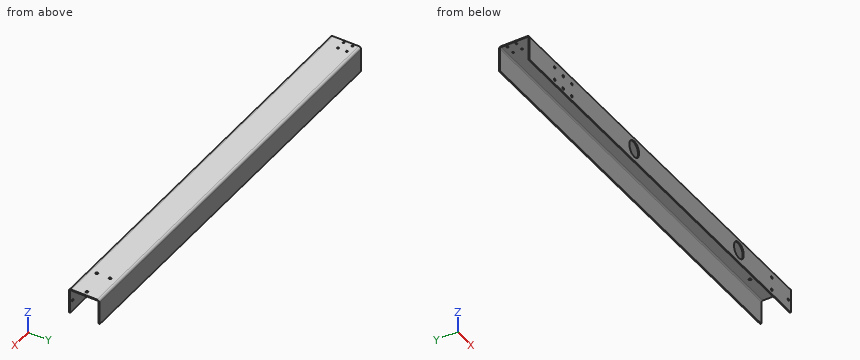
```python
from build123d import *

# Parameters (mm, degrees)
SKETCH1_W                           = 1203.325
SKETCH1_H                           = 74.6125
BASE_FLANGE1_DEPTH                  = 3.175
EDGE_FLANGE1_STRIP_W                = 20.32
EDGE_FLANGE1_STRIP_H                = 3.175
EDGE_FLANGE1_STRIP_CUT_DEPTH        = 1203.325
EDGE_FLANGE1_DEPTH                  = 1203.325
EDGE_FLANGE2_STRIP_W                = 20.32
EDGE_FLANGE2_STRIP_H                = 3.175
EDGE_FLANGE2_STRIP_CUT_DEPTH        = 1203.325
EDGE_FLANGE2_DEPTH                  = 1203.325
F_9_32_0_28125_DIAMETER_HOLE3_D     = 7.14375
F_9_32_0_28125_DIAMETER_HOLE3_DEPTH = 3.175
FILLET1_R                           = 3.175
F_9_32_0_28125_DIAMETER_HOLE1_D     = 7.14375
F_9_32_0_28125_DIAMETER_HOLE1_DEPTH = 3.175
F_9_32_0_28125_DIAMETER_HOLE2_D     = 7.14375
F_1_1_71_DOWEL_SLOT1_DEPTH          = 3.175
F_10_0_1935_DIAMETER_HOLE1_D        = 4.9149
LPATTERN2_COUNT                     = 2
LPATTERN2_PITCH                     = 25.4
LPATTERN2_COUNT_DIR2                = 2
LPATTERN2_PITCH_DIR2                = 25.4


# Read off the part's stored shape, not the designer's step: 1 (1.71) Dowel Slot1
# Sheet-metal steps are written as plain solids
with BuildPart() as part:
    # Sketch1 → Base-Flange1 (new body)
    with BuildSketch(Plane(origin=(0, 0, 0), x_dir=(1, 0, 0), z_dir=(0, 1, 0))):
        Rectangle(SKETCH1_W, SKETCH1_H)
    extrude(amount=BASE_FLANGE1_DEPTH)

    # Edge-Flange1 strip (across the edge) → Edge-Flange1 strip cut (cut)
    with BuildSketch(Plane(origin=(-601.6625, 3.175, 37.30625), x_dir=(0, 0, -1), z_dir=(1, 0, 0))):
        with Locations((-3.175, -1.5875)):
            Rectangle(EDGE_FLANGE1_STRIP_W, EDGE_FLANGE1_STRIP_H)
    extrude(amount=EDGE_FLANGE1_STRIP_CUT_DEPTH, mode=Mode.SUBTRACT)

    # Edge-Flange1 section (across the edge) → Edge-Flange1 (add)
    with BuildSketch(Plane(origin=(-601.6625, 3.175, 37.30625), x_dir=(0, 0, -1), z_dir=(1, 0, 0))):
        with BuildLine():
            Line((0, 3.81), (0, 85.725))
            Line((0, 85.725), (3.175, 85.725))
            Line((3.175, 85.725), (3.175, 3.81))
            ThreePointArc((3.175, 3.81), (4.290923164, 1.115923164), (6.985, 0))
            Line((6.985, 0), (6.985, -3.175))
            ThreePointArc((6.985, -3.175), (2.045859133, -1.129140867), (0, 3.81))
        make_face()
    extrude(amount=EDGE_FLANGE1_DEPTH)

    # Edge-Flange2 strip (across the edge) → Edge-Flange2 strip cut (cut)
    with BuildSketch(Plane(origin=(-601.6625, 88.9, 34.13125), x_dir=(0, -1, 0), z_dir=(1, 0, 0))):
        with Locations((-3.175, -1.5875)):
            Rectangle(EDGE_FLANGE2_STRIP_W, EDGE_FLANGE2_STRIP_H)
    extrude(amount=EDGE_FLANGE2_STRIP_CUT_DEPTH, mode=Mode.SUBTRACT)

    # Edge-Flange2 section (across the edge) → Edge-Flange2 (add)
    with BuildSketch(Plane(origin=(-601.6625, 88.9, 34.13125), x_dir=(0, -1, 0), z_dir=(1, 0, 0))):
        with BuildLine():
            Line((0, 3.81), (0, 71.4375))
            Line((0, 71.4375), (3.175, 71.4375))
            Line((3.175, 71.4375), (3.175, 3.81))
            ThreePointArc((3.175, 3.81), (4.290923164, 1.115923164), (6.985, 0))
            Line((6.985, 0), (6.985, -3.175))
            ThreePointArc((6.985, -3.175), (2.045859133, -1.129140867), (0, 3.81))
        make_face()
    extrude(amount=EDGE_FLANGE2_DEPTH)

    # 9/32 (0.28125) Diameter Hole3
    with Locations(Plane(origin=(0, 0, 0), x_dir=(-1, 0, 0), z_dir=(0, -1, 0))):
        with Locations((446.0875, -11.90625), (446.0875, 26.19375), (485.775, 24.60625), (485.775, -13.49375), (406.4, -13.49375), (406.4, 24.60625)):
            Hole(F_9_32_0_28125_DIAMETER_HOLE3_D / 2, depth=F_9_32_0_28125_DIAMETER_HOLE3_DEPTH)

    # Fillet1
    fillet1_edges = [part.edges().sort_by_distance(p)[0] for p in [
        (-601.6625, 87.3125, -37.30625),
        (601.6625, 87.3125, -37.30625),
        (-601.6625, 1.5875, -37.30625),
        (601.6625, 1.5875, -37.30625),
    ]]
    fillet(fillet1_edges, radius=FILLET1_R)

    # 9/32 (0.28125) Diameter Hole1
    with Locations(Plane(origin=(0, 0, 0), x_dir=(-1, 0, 0), z_dir=(0, -1, 0))):
        with Locations((-588.9625, 5.55625), (-512.7625, -13.49375), (-512.7625, 24.60625)):
            Hole(F_9_32_0_28125_DIAMETER_HOLE1_D / 2, depth=F_9_32_0_28125_DIAMETER_HOLE1_DEPTH)

    # 9/32 (0.28125) Diameter Hole2 (through all)
    with Locations(Plane.XY.offset(37.30625)):
        with Locations((588.9625, 44.45), (512.7625, 63.5), (512.7625, 25.4)):
            Hole(F_9_32_0_28125_DIAMETER_HOLE2_D / 2)

    # 1 (1.71) Dowel Slot1 outline → 1 (1.71) Dowel Slot1 (cut)
    with BuildSketch(Plane(origin=(0, 0, 0), x_dir=(1, 0, 0), z_dir=(0, 1, 0))):
        with BuildLine():
            ThreePointArc((382.87325, 3.20675), (361.15625, 24.92375), (339.43925, 3.20675))
            Line((339.43925, 3.20675), (339.43925, -1.61925))
            ThreePointArc((339.43925, -1.61925), (361.15625, -23.33625), (382.87325, -1.61925))
            Line((382.87325, -1.61925), (382.87325, 3.20675))
        make_face()
        with BuildLine():
            ThreePointArc((-98.13925, 3.20675), (-119.85625, 24.92375), (-141.57325, 3.20675))
            Line((-141.57325, 3.20675), (-141.57325, -1.61925))
            ThreePointArc((-141.57325, -1.61925), (-119.85625, -23.33625), (-98.13925, -1.61925))
            Line((-98.13925, -1.61925), (-98.13925, 3.20675))
        make_face()
    extrude(amount=F_1_1_71_DOWEL_SLOT1_DEPTH, mode=Mode.SUBTRACT)

    # #10 (0.1935) Diameter Hole1 (through all)
    with Locations(Plane.XY.offset(37.30625)):
        with Locations((-593.725, 68.2625)):
            f_10_0_1935_diameter_hole1 = Hole(F_10_0_1935_DIAMETER_HOLE1_D / 2)

    # LPattern2: 10 _0.1935_ Diameter Hole1 2 × 2
    with Locations(*[(i * LPATTERN2_PITCH, -j * LPATTERN2_PITCH_DIR2, 0) for i in range(LPATTERN2_COUNT) for j in range(LPATTERN2_COUNT_DIR2) if (i, j) != (0, 0)]):
        add(f_10_0_1935_diameter_hole1, mode=Mode.SUBTRACT)


solid = part.part
```
Can you work these out from the model? Positions are in its coordinate system, mm. Give positions to 0.01 mm unless a question says otherwise; leave off trailing zeros. Order: outer loops, then holes, each group sorted by start corner. A loop starts at its lowest first (then second) coordinate and runs counter-clockwise, first axis right, second up. Notation, with made-up numbers: M 21.25,20.5 L 78.25,20.5 A4 cw 78.25,24.5 Z; hole C -4,38 d11. An arc over 180 degrees is marked long. Write item = value, one per line. Start each with the question number.
Q1. I need wall thicknesses on probe 1 along Y at (x, z) = (-327, 30) (3 decimals); probe 2 along Z at (x, y) = (-51, 67); probe 3 along Y at (x, z) = (-73.5, 32.5). Which ranges of each line are inside material? Lowest first, please. Write a range as [from, to].
Q2. Suppose I cut it at A-A (x = -505). Write out the boundary of the cut face in (y, z) (3 decimals), plus the area to 3 significant figures.
Q3. Will these pins go through, and if not, where does the flat tip stop? pin 1 Ø5.5 at (x, z) = (-446.09, -26.19) entering from -Y (3 decimals); pin 2 Ø4.5 at (x, y) = (-568.33, 42.86) entering from -Z; pin 3 Ø1 at (x, y) = (-256.5, 15) entering from -Z.
Check result:
q1.probe_1 = [0, 3.175], [85.725, 88.9]
q1.probe_2 = [34.13, 37.31]
q1.probe_3 = [0.35, 3.86], [85.04, 88.55]
q2.outline = M 0,-37.306 L 3.175,-37.306 L 3.175,30.321 A3.81 cw 6.985,34.131 L 81.915,34.131 A3.81 cw 85.725,30.321 L 85.725,-37.306 L 88.9,-37.306 L 88.9,30.321 A6.985 ccw 81.915,37.306 L 6.985,37.306 A6.985 ccw 0,30.321 Z
q2.area = 721 mm2
q3.pin_1 = 85.725
q3.pin_2 = through
q3.pin_3 = 34.13
